Verification items for the finished model (mm, model axes). Give positions to 0.01 mm unless a question says otherwise; leave off trailing zeros. Loops run counter-clockwise (first coordinate to the right, second up) from the corner with the lowest first, then second, coordinate; pieces in that order, holes last. Notation, with made-up numbers: M -13.5,-20.5 L 14.5,-20.5 A7 cw 14.5,-13.5 Z; hole C 72.5,-28.75 d6. An arc over 180 degrees is marked long. Use CSV: the item, a comma, the result in double quotes.
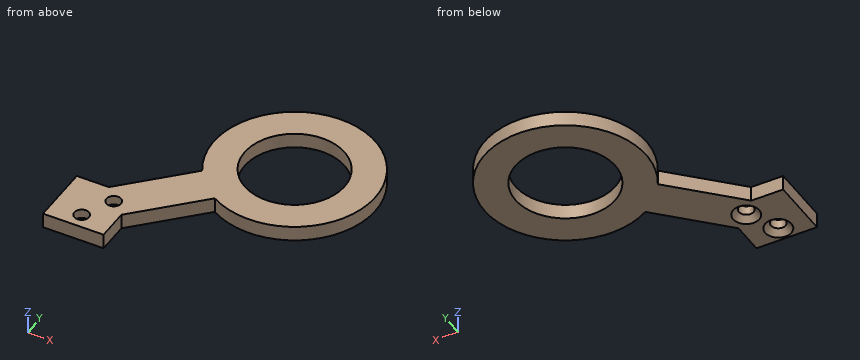
from build123d import *

# Parameters (mm, degrees)
STOP_RING_D19P76_OD32_START               = -3
SKETCH1_R                                 = 16
SKETCH1_R_2                               = 9.88
STOP_RING_D19P76_OD32_DEPTH               = 3
OUTBOARD_BRIDGE_START                     = -3
OUTBOARD_BRIDGE_DEPTH                     = 3
BASE_ATTACHMENT_PAD_START                 = -3
SKETCH3_W                                 = 12
SKETCH3_H                                 = 12
BASE_ATTACHMENT_PAD_DEPTH                 = 3
SKETCH8_R                                 = 1.45
STOP_MOUNT_D2P9_THROUGH_DEPTH             = 3.01
SKETCH9_R                                 = 2.6
STOP_MOUNT_CSK_D5P2_90DEG_DEPTH           = 1.15
STOP_MOUNT_CSK_D5P2_90DEG_DRAFT           = -45
STOP_MOUNT_CSK_D5P2_90DEG_PROFILE_2_DEPTH = 1.15
STOP_MOUNT_CSK_D5P2_90DEG_PROFILE_2_DRAFT = -45


with BuildPart() as part:
    # Sketch1 → Stop_Ring_D19p76_OD32 (new body)
    with BuildSketch(Plane.XY.offset(STOP_RING_D19P76_OD32_START)):
        with Locations((50, 50)):
            Circle(SKETCH1_R)
        with Locations((50, 50)):
            Circle(SKETCH1_R_2, mode=Mode.SUBTRACT)
    extrude(amount=STOP_RING_D19P76_OD32_DEPTH)

    # Sketch2 → Outboard_Bridge (add)
    with BuildSketch(Plane.XY.offset(OUTBOARD_BRIDGE_START)):
        Polygon((21.171572875, 26.828427125), (37.671572875, 43.328427125), (43.328427125, 37.671572875), (26.828427125, 21.171572875), align=None)
    extrude(amount=OUTBOARD_BRIDGE_DEPTH)

    # Sketch3 → Base_Attachment_Pad (add)
    with BuildSketch(Plane.XY.offset(BASE_ATTACHMENT_PAD_START)):
        with Locations((24, 24)):
            Rectangle(SKETCH3_W, SKETCH3_H)
    extrude(amount=BASE_ATTACHMENT_PAD_DEPTH)

    # Sketch8 → Stop_Mount_D2p9_Through (cut)
    with BuildSketch(Plane(origin=(0, 0, -3), x_dir=(-1, 0, 0), z_dir=(0, 0, -1))):
        with Locations((-24, 21)):
            Circle(SKETCH8_R)
        with Locations((-27, 27)):
            Circle(SKETCH8_R)
    extrude(amount=-STOP_MOUNT_D2P9_THROUGH_DEPTH, mode=Mode.SUBTRACT)


with BuildPart() as stop_mount_csk_d5p2_90deg_tool:
    # Sketch9 → Stop_Mount_CSK_D5p2_90deg (with draft: the straight prism first)
    with BuildSketch(Plane(origin=(0, 0, -3), x_dir=(-1, 0, 0), z_dir=(0, 0, -1))):
        with Locations((-24, 21)):
            Circle(SKETCH9_R)
    extrude(amount=-STOP_MOUNT_CSK_D5P2_90DEG_DEPTH)
    # Stop_Mount_CSK_D5p2_90deg: the draft: its side faces are tilted about the plane it starts from
    stop_mount_csk_d5p2_90deg_sides = [stop_mount_csk_d5p2_90deg_tool.faces().sort_by_distance(p)[0] for p in [
        (26.6, 21, -2.425),
    ]]
    draft(stop_mount_csk_d5p2_90deg_sides, Plane(origin=(0, 0, -3), x_dir=(-1, 0, 0), z_dir=(0, 0, -1)), STOP_MOUNT_CSK_D5P2_90DEG_DRAFT)


with BuildPart() as part_1:
    add(part.part)

    # Stop_Mount_CSK_D5p2_90deg: cut by stop_mount_csk_d5p2_90deg_tool
    add(stop_mount_csk_d5p2_90deg_tool.part, mode=Mode.SUBTRACT)


with BuildPart() as stop_mount_csk_d5p2_90deg_profile_2_tool:
    # Sketch9 → Stop_Mount_CSK_D5p2_90deg profile 2 (with draft: the straight prism first)
    with BuildSketch(Plane(origin=(0, 0, -3), x_dir=(-1, 0, 0), z_dir=(0, 0, -1))):
        with Locations((-27, 27)):
            Circle(SKETCH9_R)
    extrude(amount=-STOP_MOUNT_CSK_D5P2_90DEG_PROFILE_2_DEPTH)
    # Stop_Mount_CSK_D5p2_90deg profile 2: the draft: its side faces are tilted about the plane it starts from
    stop_mount_csk_d5p2_90deg_profile_2_sides = [stop_mount_csk_d5p2_90deg_profile_2_tool.faces().sort_by_distance(p)[0] for p in [
        (29.6, 27, -2.425),
    ]]
    draft(stop_mount_csk_d5p2_90deg_profile_2_sides, Plane(origin=(0, 0, -3), x_dir=(-1, 0, 0), z_dir=(0, 0, -1)), STOP_MOUNT_CSK_D5P2_90DEG_PROFILE_2_DRAFT)


with BuildPart() as part_2:
    add(part_1.part)

    # Stop_Mount_CSK_D5p2_90deg profile 2: cut by stop_mount_csk_d5p2_90deg_profile_2_tool
    add(stop_mount_csk_d5p2_90deg_profile_2_tool.part, mode=Mode.SUBTRACT)


solid = part_2.part
(1) Scan lines: L1, parallel to Y at x = 24, z = -0.75; L2, parallel to X at y = 49.5, z = -0.75; L3, parallel to Y at x = 26.5, z = -2.8. Record each from-to range of solid material in increasing order. Write a range as from..to.
Calculated:
L1,"y = 18..19.55, 22.45..30"
L2,"x = 34.01..40.13, 59.87..65.99"
L3,"y = 18..24.65, 29.35..32.16"
(2) Depth check by flat-ended pin: pin 1 Ø1 at (y, z) = (46, -1.5) entering from -X. Enter the tip coordinate at first touch or a pass-through.
Calculated:
pin 1,"stops at x = 34.39"
(3) Section check D-D on y = 27. Record the cut outline in (x, z), plus the area to 3 significant figures.
Calculated:
outline,"M 18,-3 L 24.4,-3 L 25.55,-1.85 L 25.55,0 L 18,0 Z; M 28.45,-1.85 L 29.6,-3 L 32.66,-3 L 32.66,0 L 28.45,0 Z"
area,"33.9 mm²"
(4) Section check A-A on y = 50. Record the cut outline in (x, z).
Calculated:
outline,"M 34,-3 L 40.12,-3 L 40.12,0 L 34,0 Z; M 59.88,-3 L 66,-3 L 66,0 L 59.88,0 Z"
(5) Section check C-C on z = -0.7. Record the cut outline in (x, y), plus the area to 3 significant figures.
Calculated:
outline,"M 18,18 L 30,18 L 30,24.34 L 41.87,36.22 A16 ccw long 36.22,41.87 L 24.34,30 L 18,30 Z; hole C 24,21 d2.9; hole C 27,27 d2.9; hole C 50,50 d19.76"
area,"744 mm²"
